from build123d import *

# Parameters (mm, degrees)
F0_W           = 126.4
F0_H           = 152.4
F0_W_2         = 124
F0_H_2         = 150
F1_DEPTH       = 10.2
F2_DEPTH       = 1.2
F3_R           = 2
F4_R           = 1.5
F5_DEPTH       = 9.2
F6_D           = 3
F6_CBORE_D     = 4
F6_CBORE_DEPTH = 1.2
F7_R           = 3
F7_R_2         = 1.375
F8_DEPTH       = 6.7
F7_R_3         = 0.4
F9_DEPTH       = 5


# Not quite as in the source:
# - a feature names something its author has since deleted; it is built from what else it names


with BuildPart() as f1:
    # F0 (on Top) → F1 (new body)
    with BuildSketch(Plane.XY):
        Rectangle(F0_W, F0_H)
        Rectangle(F0_W_2, F0_H_2, mode=Mode.SUBTRACT)
    extrude(amount=F1_DEPTH)

    # F0 (on Top) → F2 (join)
    with BuildSketch(Plane.XY):
        Rectangle(F0_W_2, F0_H_2)
    extrude(amount=F2_DEPTH)

    # F3
    f3_edges = [f1.edges().sort_by_distance(p)[0] for p in [
        (63.2, -76.2, 5.1),
        (-63.2, 76.2, 5.1),
        (63.2, 76.2, 5.1),
        (-63.2, -76.2, 5.1),
    ]]
    fillet(f3_edges, radius=F3_R)

    # F4 (on face) → F5 (join)
    with BuildSketch(Plane(origin=(0, 0, 0), x_dir=(1, 0, 0), z_dir=(0, 0, -1))):
        with BuildLine():
            Line((62, 69), (62, 75))
            Line((62, 75), (56, 75))
            Line((56, 75), (56, 72))
            ThreePointArc((56, 72), (56.8786796564, 69.8786796564), (59, 69))
            Line((59, 69), (62, 69))
        make_face()
        with Locations((59, 72)):
            Circle(F4_R, mode=Mode.SUBTRACT)
        with Locations((59, 72)):
            Circle(F4_R)
        with BuildLine():
            Line((-56, 75), (-62, 75))
            Line((-62, 75), (-62, 69))
            Line((-62, 69), (-59, 69))
            ThreePointArc((-59, 69), (-56.8786796564, 69.8786796564), (-56, 72))
            Line((-56, 72), (-56, 75))
        make_face()
        with Locations((-59, 72)):
            Circle(F4_R, mode=Mode.SUBTRACT)
        with Locations((-59, 72)):
            Circle(F4_R)
    extrude(amount=-F5_DEPTH)

    # F6 (through all)
    with Locations(Plane(origin=(0, 0, 0), x_dir=(1, 0, 0), z_dir=(0, 0, -1))):
        with Locations((59, 72), (-59, 72)):
            CounterBoreHole(F6_D / 2, F6_CBORE_D / 2, F6_CBORE_DEPTH)

    # F7 (on face) → F8 (join)
    with BuildSketch(Plane.XY.offset(1.2)):
        with Locations((55.0223472919, -16.0672999918)):
            Circle(F7_R)
        with Locations((55.0223472919, -16.0672999918)):
            Circle(F7_R_2, mode=Mode.SUBTRACT)
        with Locations((-2.9776527081, -16.0672999918)):
            Circle(F7_R)
        with Locations((-2.9776527081, -16.0672999918)):
            Circle(F7_R_2, mode=Mode.SUBTRACT)
        with Locations((-2.9776527081, -65.0672999918)):
            Circle(F7_R)
        with Locations((-2.9776527081, -65.0672999918)):
            Circle(F7_R_2, mode=Mode.SUBTRACT)
        with Locations((55.0223472919, -65.0672999918)):
            Circle(F7_R)
        with Locations((55.0223472919, -65.0672999918)):
            Circle(F7_R_2, mode=Mode.SUBTRACT)
    extrude(amount=F8_DEPTH)

    # F7 (on face) → F9 (join)
    with BuildSketch(Plane.XY.offset(1.2)):
        with Locations((-57.0500735752, 2.4133773954)):
            Circle(F7_R_3)
    extrude(amount=F9_DEPTH)


solid = f1.part
Can you work these out from the model? Positions are in its coordinate system, mm. A direction names the side the tool comes from. Give positions to 0.01 mm unless a question says otherwise; leave off trailing zeros. Loops run counter-clockwise (first coordinate to the right, second up) from the corner with the lowest first, then second, coordinate; pieces in that order, holes last. Notation, with made-up numbers: (30.5, -0.5) -> (56.5, -0.5) arc R11 ccw to (56.5, 10.5) -> close; hole circle Ø3 at (39.5, 45). An arc over 180 degrees is marked (long way). Write item = value, one per line.
1) Suppose I cut it at A-A on x = -42. Write out the boundary of the cut face in (y, z).
Check result:
outline = (-76.2, 0) -> (76.2, 0) -> (76.2, 10.2) -> (75, 10.2) -> (75, 1.2) -> (-75, 1.2) -> (-75, 10.2) -> (-76.2, 10.2) -> close
2) Thinking about a two-plate mould opening in X: for faces 1 (the flat face through (60.3, -73.4, 9.2)), 2 (the flat face through (63.2, -1, 5)), 3 (the flat face through (-63.2, -1, 5)), which applies, released by +X, released by -X, zero draft, split by the parting line, or undercut?
Check result:
face_1 = undercut
face_2 = released by +X
face_3 = released by -X
3) I need wall thicknesses on L1, parallel to X at y = -52, z = 5; L2, parallel to X at y = -72, z = 0.55; L3, parallel to Y at x = 24.5, z = 9. Which ranges of each line are inside material? Lowest first, please. Write a range as from..to.
Check result:
L1 = -63.2..-62, 62..63.2
L2 = -63.2..-61, -57..57, 61..63.2
L3 = -76.2..-75, 75..76.2
4) For faces 4 (the flat face through (-56, -73, 5)), 5 (the cylindrical face through (-57.925, -73.686, 0.592)), which set-ups out of +Z, -Z, +X, -X, +Y, -Y let a thin tool reach every point of the face, with its end or its side?
Check result:
face_4 = +Z
face_5 = -Z
5) Will these pins go through, and if not, where does the flat tip stop? pin 1 (5 mm diameter, centred on x = -2, y = -17, fed in from +Z); pin 2 (5 mm diameter, centred on x = 59, y = -72, fed in from -Z); pin 3 (3 mm diameter, centred on x = 59.5, y = -72, fed in from +Z); pin 4 (1.4 mm diameter, centred on x = -2.5, y = -16, fed in from +Z).
Check result:
pin_1 = 7.9
pin_2 = 0
pin_3 = 9.2
pin_4 = 1.2
6) Suppose I cut it at B-B on y = 60. Write out the boundary of the cut face in (x, z).
Check result:
outline = (-63.2, 0) -> (63.2, 0) -> (63.2, 10.2) -> (62, 10.2) -> (62, 1.2) -> (-62, 1.2) -> (-62, 10.2) -> (-63.2, 10.2) -> close
